from build123d import *

# Parameters (mm, degrees)
SKETCH1_W           = 10.2
SKETCH1_H           = 16.8
SKETCH1_W_2         = 6.2
SKETCH1_H_2         = 14.1
BOSS_EXTRUDE1_DEPTH = 3
SKETCH2_W           = 6.2
SKETCH2_H           = 2
CUT_EXTRUDE1_DEPTH  = 25.4
SKETCH3_W           = 10.2
SKETCH3_H           = 16.8
BOSS_EXTRUDE2_DEPTH = 2
SKETCH4_R           = 14
SKETCH4_R_2         = 12
BOSS_EXTRUDE4_DEPTH = 5
BOSS_EXTRUDE5_START = 2.54
SKETCH5_R           = 14
BOSS_EXTRUDE5_DEPTH = 2.54
SKETCH6_W           = 6.2
SKETCH6_H           = 3
CUT_EXTRUDE2_DEPTH  = 7.62
FILLET1_R           = 2


with BuildPart() as part:
    # Sketch1 → Boss-Extrude1 (new body)
    with BuildSketch(Plane(origin=(0, 0, 0), x_dir=(1, 0, 0), z_dir=(0, 1, 0))):
        with Locations((-29.627149571, -6.071905286)):
            Rectangle(SKETCH1_W, SKETCH1_H)
        with Locations((-29.627149571, -5.421905286)):
            Rectangle(SKETCH1_W_2, SKETCH1_H_2, mode=Mode.SUBTRACT)
    extrude(amount=BOSS_EXTRUDE1_DEPTH)

    # Sketch2 → Cut-Extrude1 (cut)
    with BuildSketch(Plane.XY.offset(14.471905286)):
        with Locations((-29.627149571, 2)):
            Rectangle(SKETCH2_W, SKETCH2_H)
    extrude(amount=-CUT_EXTRUDE1_DEPTH, mode=Mode.SUBTRACT)

    # Sketch3 → Boss-Extrude2 (add)
    with BuildSketch(Plane.XZ):
        with Locations((-29.627149571, 6.071905286)):
            Rectangle(SKETCH3_W, SKETCH3_H)
    extrude(amount=BOSS_EXTRUDE2_DEPTH)

    # Sketch4 → Boss-Extrude4 (add)
    with BuildSketch(Plane.XZ.offset(2)):
        with Locations(Location((-29.627149571, 3.222245286, 0), (0, 0, 270))):
            Circle(SKETCH4_R)
        with Locations((-29.627149571, 3.222245286)):
            Circle(SKETCH4_R_2, mode=Mode.SUBTRACT)
    extrude(amount=-BOSS_EXTRUDE4_DEPTH)

    # Sketch5 → Boss-Extrude5 (add)
    with BuildSketch(Plane.XZ.offset(2).offset(BOSS_EXTRUDE5_START)):
        with Locations(Location((-29.627149571, 3.222245286, 0), (0, 0, 270))):
            Circle(SKETCH5_R)
    extrude(amount=-BOSS_EXTRUDE5_DEPTH)

    # Sketch6 → Cut-Extrude2 (cut)
    with BuildSketch(Plane.XY.offset(14.471905286)):
        with Locations((-29.627149571, 1.5)):
            Rectangle(SKETCH6_W, SKETCH6_H)
    extrude(amount=CUT_EXTRUDE2_DEPTH, mode=Mode.SUBTRACT)

    # Fillet1
    fillet1_edges = [part.edges().sort_by_distance(p)[0] for p in [
        (-29.627149571, -4.54, 17.222245286),
    ]]
    fillet(fillet1_edges, radius=FILLET1_R)


solid = part.part
The model under review builds one solid part; all positions refer to its coordinate system, in mm. A direction names the side the tool comes from. Give positions to 0.01 mm unless a question says otherwise; leave off trailing zeros. Order: outer loops, then holes, each group sorted by start corner. A loop starts at its lowest first (then second) coordinate and runs counter-clockwise, first axis right, second up. Notation, with made-up numbers: (21, 34.5) -> (61, 34.5) arc R10 ccw to (61, 41.5) -> close; hole circle Ø1 at (9.25, 14). An arc over 180 degrees is marked (long way). Write item = value, one per line. Start each with the question number.
(1) Take a section at A-A (y = 1.5). Write out the cut boundary in (x, z), plus the area to 3 significant figures.
(2) Tool access review of faces 4 (the flat face through (-30, 0, 16)), 5 (the flat face through (-30, 0, -2.328)): name each direction out of +Z, -Z, +X, -X, +Y, -Y from which nothing blocks a thin tool from reaching the whole face with its end or side.
(3) For pin 1 Ø1 at (x, z) = (-36, -0.5) entering from +Y; pin 2 Ø0.6 at (x, z) = (-30, 15) entering from +Y; pin 3 Ø1 at (y, z) = (1.5, 16) entering from +X, all flat-tipped, find the tip position at first contact; note any pin that passes through.
(4) Take a section at B-B (y = -3). Write out the cut boundary in (x, z).
(5) Draft analysis for pull direction X (two halves, no side actions). For faces 1 (the flat face through (-29, -4.54, 3)), 2 (the cylindrical face through (-34.99, 0.19, -9.71)), 3 (the flat face through (-30, 0, 14.472)), state which applies: +X half, -X half, draft (parallel to the pull), parting line (faces both ways), or undercut.
(6) For L1, parallel to X at y = 0.75, z = 0.75; L2, parallel to Y at x = -24.5, z = -4; L3, parallel to Z at x = -38.75, y = -1.25, list the stretches that pass through material, from the lowest coordinate up. Write a range as from..to.
Returned:
q1.outline = (-34.73, -2.33) -> (-32.73, -2.33) -> (-32.73, 14.47) -> (-33.8, 14.47) arc R12 cw to (-32.73, 14.81) -> (-32.73, 16.87) arc R14 ccw (long way) to (-26.53, 16.87) -> (-26.53, 14.81) arc R12 cw to (-25.45, 14.47) -> (-26.53, 14.47) -> (-26.53, -2.33) -> (-24.53, -2.33) -> (-24.53, 14.08) arc R12 cw (long way) to (-34.73, 14.08) -> close
q1.area = 218 mm²
q2.face_4 = +Z, +Y
q2.face_5 = +Y
q3.pin_1 = -2
q3.pin_2 = 0
q3.pin_3 = -22.9
q4.outline = circle Ø27.89 at (-29.63, 3.22)
q5.face_1 = draft
q5.face_2 = parting line
q5.face_3 = undercut
q6.L1 = -43.41..-41.37, -34.73..-32.73, -26.53..-24.53, -17.88..-15.85
q6.L2 = -4.54..-2
q6.L3 = -7.4..-4.57, 11.02..13.84
